Autodesk Inventor part; units mm, degrees
ref_plane "YZ Plane" through (0, 0, 0) normal (1, 0, 0) x (0, 1, 0)
ref_plane "XZ Plane" through (0, 0, 0) normal (0, 1, 0) x (-1, 0, 0)
ref_plane "XY Plane" through (0, 0, 0) normal (0, 0, 1) x (1, 0, 0)
sketch "Sketch1" plane through (0, 0, 0) normal (1, 0, 0) x (0, 1, 0)
  arc A0 (2.8, 0) -> (2.5667, 0.7739) centre (1.4, 0) ccw
  line L0 (0, 7.7385) -> (0, -8.1997) construction
  line L1 (-1.7375, 0) -> (6.7594, 0) construction
  line L2 (0, 3.5) -> (1.93, 2.2938)
  line L3 (2.4, 1.4458) -> (2.4, 1.3266)
  arc A1 (2.4, 1.4458) -> (1.93, 2.2938) centre (1.4, 1.4458) ccw
  line L4 (0, 3.5) -> (0, 7)
  line L5 (0, 7) -> (2.4, 7)
  line L6 (3.4, 6) -> (3.4, 0)
  arc A2 (3.4, 6) -> (2.4, 7) centre (2.4, 6) ccw
  arc A3 (2.4, 1.3266) -> (2.5667, 0.7739) centre (3.4, 1.3266) ccw
  arc A4 (2.5667, -0.7739) -> (2.8, 0) centre (1.4, 0) ccw
  line L7 (0, -3.5) -> (1.93, -2.2938)
  line L8 (2.4, -1.4458) -> (2.4, -1.3266)
  arc A5 (1.93, -2.2938) -> (2.4, -1.4458) centre (1.4, -1.4458) ccw
  line L9 (0, -3.5) -> (0, -7)
  line L10 (0, -7) -> (2.4, -7)
  line L11 (3.4, -6) -> (3.4, 0)
  arc A6 (2.4, -7) -> (3.4, -6) centre (2.4, -6) ccw
  arc A7 (2.5667, -0.7739) -> (2.4, -1.3266) centre (3.4, -1.3266) ccw
  point P0 (0, 0)
  point P1 (2.4, 2)
  point P2 (2.4, 0.9798)
  point P3 (3.4, 7)
  point P4 (0, -7.7385)
  dimension "d0" = 2.8
  dimension "d1" = 1
  dimension "d2" = 3.5
  dimension "d3" = 2
  dimension "d4" = 1
  dimension "d5" = 7
  dimension "d6" = 2
  dimension "d7" = 7
  dimension "d8" = 1
  dimension "d9" = 1
extrude "Extrusion1" add sketch "Sketch1" along normal blind 3.5
sketch "Sketch2" plane through (0, 3.4, 6) normal (0, 1, 0) x (1, 0, 0)
  line L0 (0, 6) -> (3.5416, 6) construction
  line L1 (0, -1) -> (3.5, -1)
  line L2 (1.75, -1) -> (1.75, 12.2689) construction
  point P0 (1.75, 0.775)
  point P1 (1.75, 11.225)
  dimension "d12" = 5.225
hole "Hole1" at (1.75, 3.4, 5.225) at (1.75, 3.4, -5.225) direction (0, -1, 0) diameter 1.5 end through all counterbore diameter 2.5 counterbore depth 1.3
fillet "Fillet1" radius 1 2 edges at (1.75, 0, 3.5) (1.75, 0, -3.5)
properties part number "3rd_phalanx_fingertip_holer"
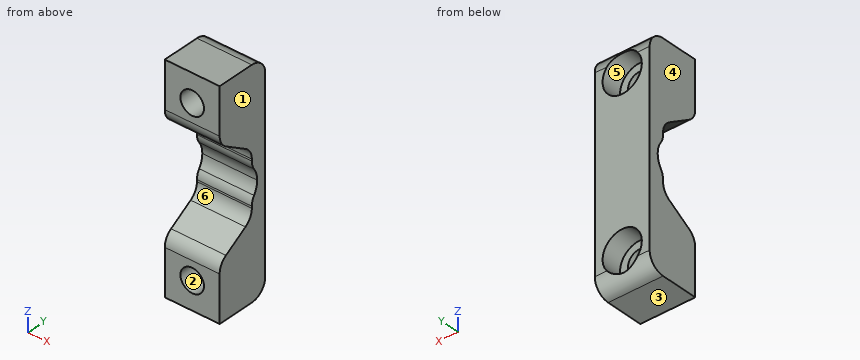
Read the model definition and answer for the solid it produces. Units are mm, in the model's axes. Face numbers are marked on the shaded views. A direction names the side the tool comes from. Coordinates: 2 decimals unless noted, no trailing zeros. Write each loop counter-clockwise with the first axis right and the second up, starting at its lowest first coordinate (ties: lowest second). Pieces come first, ordered by that corner, then holes. Notation, with made-up numbers: (71.25, 26.25) - (91.25, 26.25) arc R6 ccw to (91.25, 31.25) - close; hole circle Ø6 at (0, 53.25). An arc over 180 degrees is marked (long way). One line per question, with ' | ' between items.
Q1. Find section B-B, the plane x = 0.35. Write down the section's boundary in (y, z), plus the area to 3 significant figures.
Result set:
outline: (0, -7) - (2.4, -7) arc R1 ccw to (3.4, -6) - (3.4, 6) arc R1 ccw to (2.4, 7) - (0, 7) - (0, 4.05) arc R1 ccw to (0.47, 3.21) - (1.93, 2.29) arc R1 cw to (2.4, 1.45) - (2.4, 1.33) arc R1 ccw to (2.57, 0.77) arc R1.4 cw to (2.8, 0) arc R1.4 cw to (2.57, -0.77) arc R1 ccw to (2.4, -1.33) - (2.4, -1.45) arc R1 cw to (1.93, -2.29) - (0.47, -3.21) arc R1 ccw to (0, -4.05) - close | area: 33.4 mm^2
Q2. For the marked faces 4, 5 and 6, determine the directions among +Z, -Z, +X, -X, +Y, -Y from which every point of the face is accessible in a straight line to the end or side of a thin tool.
Result set:
face 4: +Z, -Z, -X, +Y, -Y | face 5: +Y | face 6: +X, -X, -Y
Q3. Each of these flat-tipped pins is pushed along its axis until it touches: P1, Ø1, axis at x = 2, y = 3, coming from the -Z side (3 decimals); P2, Ø1.2, axis at x = 1.5, z = 5, coming from the +Y side. Where does it stop, or does it pass through?
Result set:
P1: z = -6.995 | P2: y = 2.1
Q4. Find section C-C, the plane y = 3. Write down the section's boundary in (x, z) (3 decimals).
Result set:
outline: (0, -6.8) - (3.5, -6.8) - (3.5, 6.8) - (0, 6.8) - close; hole circle Ø2.5 at (1.75, -5.225); hole circle Ø2.5 at (1.75, 5.225)
Q5. Consider L1, parallel to Z at x = 1.75, y = 3 (3 decimals); L2, parallel to Z at x = 1.75, y = 2.9 (3 decimals); L3, parallel to Z at x = 1.75, y = 0.7 (3 decimals). Determine where each line is inside the solid, lowest interval first. Write a range as [from, to].
Result set:
L1: [-6.8, -6.475], [-3.975, 3.975], [6.475, 6.8] | L2: [-6.866, -6.475], [-3.975, 3.975], [6.475, 6.866] | L3: [-7, -5.975], [-4.475, -3.063], [3.063, 4.475], [5.975, 7]
Q6. Find section D-D, the plane x = 2. State how many separate pieces and enclosed holes the cut face has, plus the area to 3 significant figures.
Result set:
separate pieces: 3 | enclosed holes: 0 | area: 21.1 mm^2
Q7. Determine the mould class of the marked faces 1, 2 and 3 for opening direction X: +X half, -X half, draft (parallel to the pull), parting line (faces both ways), or undercut.
Result set:
face 1: +X half | face 2: undercut | face 3: draft
Q8. Find section A-A, the plane y = 1.7. Write down the section's boundary in (x, z) (3 decimals).
Result set:
outline: (0, -7) - (3.5, -7) - (3.5, -2.438) - (0, -2.438) - close; (0, 2.438) - (3.5, 2.438) - (3.5, 7) - (0, 7) - close; hole circle Ø1.5 at (1.75, -5.225); hole circle Ø1.5 at (1.75, 5.225)
